The listing builds one solid part. Answer for the finished solid, in the listing's coordinates (mm). Face numbers are marked on the shaded views. A direction names the side the tool comes from. Give positions to 0.01 mm unless a question says otherwise; leave off trailing zeros. Loops run counter-clockwise (first coordinate to the right, second up) from the corner with the lowest first, then second, coordinate; pieces in that order, holes last. Notation, with made-up numbers: (-36, -12) - (-20, -12) arc R16 cw to (-20, 17) - close; hole circle Ø9 at (70.25, 40). An arc over 180 degrees is marked (long way). Answer as CSV lines item,"result". Start each with the question number.
1) A cutting plane is placed at B-B (x = 77). Determine the outline of the cut face in (y, z) (3 decimals).
2) A cutting plane is placed at C-C (y = 31.5). Determine the outline of the cut face in (x, z) (3 decimals), and give its area (3 significant figures).
3) A cutting plane is placed at A-A (z = 1.5). Determine the outline of the cut face in (x, y) (3 decimals).
4) For the marked faces 5, 6, 7 and 8, determine the directions among +Z, -Z, +X, -X, +Y, -Y from which every point of the face is accessible in a straight line to the end or side of a thin tool.
5) Flat-ended cylindrical pins translate along their axes: pin 1 (6 mm diameter, centred on x = -15, z = 16, fed in from +Y); pin 2 (16.5 mm diameter, centred on x = -1.5, y = 26.5, fed in from +Z) (3 decimals); pin 3 (5 mm diameter, centred on y = -15, z = 17, fed in from -X) (3 decimals); pin 4 (5 mm diameter, centred on y = 28.5, z = 45.5, fed in from -X). Find the tip coordinate at first contact, or state that the pin passes through.
6) Find the intervals of material crossed by line 1 along Z through (x, y) = (-33, 42.5) (3 decimals); line 2 along Y through (x, z) = (22.5, 27); line 3 along Z through (x, y) = (78, 9) (3 decimals), in increasing order.
7) For a pull along X with two mould halves and no side action, classify the marked faces 1, 2, 3 and 4 as pulls with the +X half, pulls with the -X half, needs draft (parallel to the pull), parting line crosses it, or undercut.
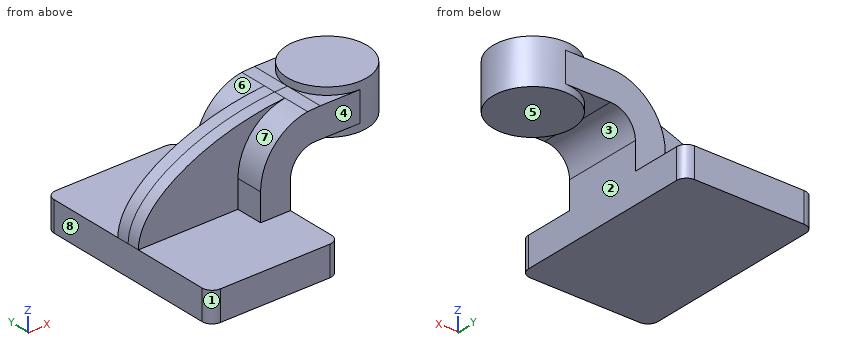
```python
from build123d import *

# Parameters (mm, degrees)
F1_DEPTH = 63.5
F2_DEPTH = 25.4
F3_DEPTH = 7.9375
F0_W     = 25.4
F0_H     = 19.05
F4_DEPTH = 25.4
F6_R     = 6.35


with BuildPart() as f1:
    # F0 (on Front) → F1 (new body, symmetric)
    with BuildSketch(Plane.XZ):
        Polygon((-41.275, 9.525), (-41.275, -9.525), (41.275, -9.525), (41.275, 9.525), (22.225, 9.525), align=None)
    extrude(amount=F1_DEPTH, both=True)

    # F0 (on Front) → F2 (join, symmetric)
    with BuildSketch(Plane.XZ):
        with BuildLine():
            Line((22.225, 9.525), (41.275, 9.525))
            Line((41.275, 9.525), (41.275, 27.0002))
            ThreePointArc((41.275, 27.0002), (45.92468, 38.22552), (57.15, 42.8752))
            Line((57.15, 42.8752), (60.325, 42.8752))
            Line((60.325, 42.8752), (60.325, 61.9252))
            add(Edge.make_bspline(
                [(52.205815, 61.573465), (54.9122, 61.753284), (57.621454, 61.871383), (60.325, 61.9252)],
                knots=[108.111477, 108.111477, 108.111477, 108.111477, 114.316845, 114.316845, 114.316845, 114.316845], degree=3))
            ThreePointArc((52.205815, 61.573465), (30.764101, 49.881196), (22.225, 27.0002))
            Line((22.225, 27.0002), (22.225, 9.525))
        make_face()
    extrude(amount=F2_DEPTH, both=True)

    # F0 (on Front) → F3 (join, symmetric)
    with BuildSketch(Plane.XZ):
        with BuildLine():
            add(Edge.make_bspline(
                [(-41.275, 9.525), (-41.22588, 36.57363), (5.054491, 58.440611), (52.205815, 61.573465)],
                knots=[0, 0, 0, 0, 108.111477, 108.111477, 108.111477, 108.111477], degree=3))
            Line((-41.275, 9.525), (22.225, 9.525))
            Line((22.225, 9.525), (22.225, 27.0002))
            ThreePointArc((22.225, 27.0002), (30.764101, 49.881196), (52.205815, 61.573465))
        make_face()
    extrude(amount=F3_DEPTH, both=True)

    # F0 (on Front) → F4 (join, symmetric)
    with BuildSketch(Plane.XZ):
        with Locations((73.025, 52.4002)):
            Rectangle(F0_W, F0_H)
    extrude(amount=F4_DEPTH, both=True)

    # F0 (on Front) → F5 (revolve)
    with BuildSketch(Plane.XZ):
        Polygon((85.725, 66.675), (85.725, 61.9252), (85.725, 42.8752), (85.725, 38.1), (111.125, 38.1), (111.125, 66.675), align=None)
    revolve(axis=Axis((85.725, 0, 52.3875), (0, 0, 1)))

    # F6
    f6_edges = [f1.edges().sort_by_distance(p)[0] for p in [
        (41.275, -63.5, 0),
        (-41.275, -63.5, 0),
        (41.275, 63.5, 0),
        (-41.275, 63.5, 0),
    ]]
    fillet(f6_edges, radius=F6_R)


solid = f1.part
```
Ans:
1,outline,"(-25.4, 42.875) - (-23.854, 42.875) - (-23.854, 38.1) - (23.854, 38.1) - (23.854, 42.875) - (25.4, 42.875) - (25.4, 61.925) - (23.854, 61.925) - (23.854, 66.675) - (-23.854, 66.675) - (-23.854, 61.925) - (-25.4, 61.925) - close"
2,outline,"(-41.275, -9.525) - (41.275, -9.525) - (41.275, 9.525) - (-41.275, 9.525) - close"
2,area,"1,570 mm2"
3,outline,"(-41.275, -57.15) arc R6.35 ccw to (-34.925, -63.5) - (34.925, -63.5) arc R6.35 ccw to (41.275, -57.15) - (41.275, 57.15) arc R6.35 ccw to (34.925, 63.5) - (-34.925, 63.5) arc R6.35 ccw to (-41.275, 57.15) - close"
4,face 5,"-Z, +X, +Y, -Y"
4,face 6,"+Z, -X, +Y"
4,face 7,"+Z, -X, -Y"
4,face 8,"+Z, -Z, -X, +Y, -Y"
5,pin 1,"y = 7.94"
5,pin 2,"z = 9.525"
5,pin 3,"x = 22.225"
5,pin 4,"through"
6,line 1,"-9.525 to 9.525"
6,line 2,"-25.4 to 25.4"
6,line 3,"38.1 to 66.675"
7,face 1,"pulls with the -X half"
7,face 2,"pulls with the +X half"
7,face 3,"undercut"
7,face 4,"needs draft"
